from build123d import *

# Parameters (mm, degrees)
BOSS_EXTRUDE1_DEPTH       = 15
CHAMFER1_SIZE             = 2.5
SKETCH2_R                 = 1.4
CUT_EXTRUDE1_DEPTH        = 41.512038564
F_3_0MM_DOWEL_HOLE1_D     = 3
F_3_0MM_DOWEL_HOLE1_DEPTH = 31.098709071
F_3_0MM_DOWEL_HOLE1_TIP   = 0.901290929


with BuildPart() as part:
    # Sketch1 → Boss-Extrude1 (new body)
    with BuildSketch(Plane.XY):
        with BuildLine():
            Line((-18.574175621, -4), (-33.574175621, -4))
            Line((-33.574175621, -4), (-33.574175621, -21))
            Line((-33.574175621, -21), (33.574175621, -21))
            Line((33.574175621, -21), (33.574175621, -4))
            Line((33.574175621, -4), (18.574175621, -4))
            ThreePointArc((18.574175621, -4), (0, -19), (-18.574175621, -4))
        make_face()
    extrude(amount=BOSS_EXTRUDE1_DEPTH)

    # Chamfer1
    chamfer1_edges = [part.edges().sort_by_distance(p)[0] for p in [
        (-33.574175621, -12.5, 15),
        (33.574175621, -12.5, 15),
        (-33.574175621, -12.5, 0),
        (33.574175621, -12.5, 0),
    ]]
    chamfer(chamfer1_edges, length=CHAMFER1_SIZE)

    # Sketch2 → Cut-Extrude1 (cut, through all)
    with BuildSketch(Plane(origin=(0, -4, 0), x_dir=(1, 0, 0), z_dir=(0, 1, 0))):
        with Locations(Location((28.441617262, -7.5, 0), (0, 0, 180))):
            Circle(SKETCH2_R)
        with Locations((-28.441617262, -7.5)):
            Circle(SKETCH2_R)
    extrude(amount=-CUT_EXTRUDE1_DEPTH, mode=Mode.SUBTRACT)

    # Ø3.0mm Dowel Hole1
    with Locations(Plane(origin=(0, -4, 0), x_dir=(1, 0, 0), z_dir=(0, 1, 0))):
        with Locations((-28.441617262, -7.5), (28.441617262, -7.5)):
            Hole(F_3_0MM_DOWEL_HOLE1_D / 2, depth=F_3_0MM_DOWEL_HOLE1_DEPTH)
            with Locations((0, 0, -(F_3_0MM_DOWEL_HOLE1_DEPTH + F_3_0MM_DOWEL_HOLE1_TIP / 2))):  # 118° drill point
                Cone(0, F_3_0MM_DOWEL_HOLE1_D / 2, F_3_0MM_DOWEL_HOLE1_TIP, mode=Mode.SUBTRACT)


solid = part.part
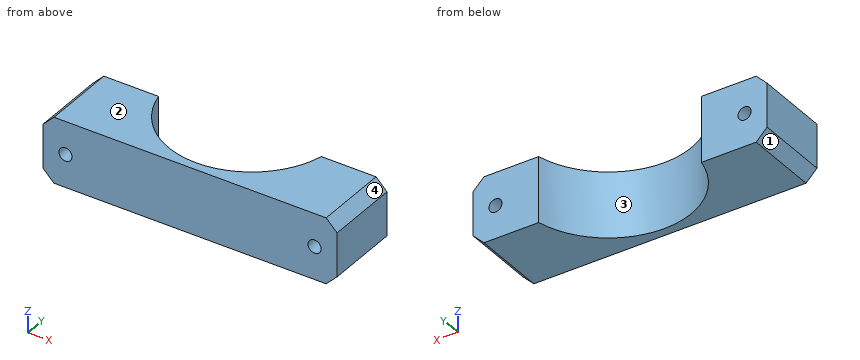
Design review of the part built by this model. Coordinates are the model's own, in mm. Face numbers are marked on the shaded views. Round coordinates to 2 decimals unless told otherwise and drop trailing zeros. Loops run counter-clockwise (first coordinate to the right, second up) from the corner with the lowest first, then second, coordinate; pieces in that order, holes last. Notation, with made-up numbers: M 10,66 L 28,66 A13 ccw 28,72 Z; hole C -0.5,-11.75 d1. An arc over 180 degrees is marked long. Answer as a JSON object with one key per item and string values.
Item 1: We need section D-D on y = -16.25. Give the boundary of the cut face in (x, z), and give its area (3 significant figures).
Answer sheet:
{"outline": "M -33.57,2.5 L -31.07,0 L -9.85,0 L -9.85,15 L -31.07,15 L -33.57,12.5 Z; M 9.85,0 L 31.07,0 L 33.57,2.5 L 33.57,12.5 L 31.07,15 L 9.85,15 Z; hole C -28.44,7.5 d3; hole C 28.44,7.5 d3", "area": "685 mm^2"}
Item 2: Wall thickness on L1, parallel to X at y = -14.5, z = 7.5; L2, parallel to X at y = -16.5, z = 7.5; L3, parallel to X at y = -15, z = 9.5: over which ranges is each line inside the solid? List them lowest first. Write a range as from..to.
Answer sheet:
{"L1": "x = -33.57..-29.94, -26.94..-12.28, 12.28..26.94, 29.94..33.57", "L2": "x = -33.57..-29.94, -26.94..-9.42, 9.42..26.94, 29.94..33.57", "L3": "x = -33.57..-11.66, 11.66..33.57"}
Item 3: We need section B-B on z = 7.5. Give the boundary of the cut face in (x, y), and give its area (3 significant figures).
Answer sheet:
{"outline": "M -33.57,-21 L -29.94,-21 L -29.94,-4 L -33.57,-4 Z; M -26.94,-21 L 26.94,-21 L 26.94,-4 L 18.57,-4 A19 cw -18.57,-4 L -26.94,-4 Z; M 29.94,-21 L 33.57,-21 L 33.57,-4 L 29.94,-4 Z", "area": "623 mm^2"}
Item 4: We need section C-C on z = 10. Give the boundary of the cut face in (x, y).
Answer sheet:
{"outline": "M -33.57,-21 L 33.57,-21 L 33.57,-4 L 18.57,-4 A19 cw -18.57,-4 L -33.57,-4 Z"}
Item 5: The part is to be moulded in two halves that separate along X. For the marked faces 1, 2, 3 and 4, say which applies: pulls with the +X half, pulls with the -X half, needs draft (parallel to the pull), parting line crosses it, or undercut.
Answer sheet:
{"face 1": "pulls with the -X half", "face 2": "needs draft", "face 3": "undercut", "face 4": "pulls with the +X half"}
Item 6: We need section A-A on y = -6. Give the boundary of the cut face in (x, z).
Answer sheet:
{"outline": "M -33.57,2.5 L -31.07,0 L -18.03,0 L -18.03,15 L -31.07,15 L -33.57,12.5 Z; M 18.03,0 L 31.07,0 L 33.57,2.5 L 33.57,12.5 L 31.07,15 L 18.03,15 Z; hole C -28.44,7.5 d3; hole C 28.44,7.5 d3"}
Item 7: Clearance check with flat-ended pins moving along their axes: P1, Ø5, axis at x = -4.5, y = -14, coming from the -Z side; P2, Ø6, axis at x = -6.5, z = 4, coming from the +Y side; P3, Ø1.5, axis at x = 6, z = 7, coming from the +Y side. State where each tip first meets the part, or that it passes through.
Answer sheet:
{"P1": "passes through", "P2": "stops at y = -16.45", "P3": "stops at y = -17.76"}
